Geometry: final body of the model. Coordinates: model frame, mm. Face numbers are marked on the shaded views. A direction names the side the tool comes from. Give positions to 0.01 mm unless a question says otherwise; leave off trailing zeros. Order: outer loops, then holes, each group sorted by start corner. A loop starts at its lowest first (then second) coordinate and runs counter-clockwise, first axis right, second up. Notation, with made-up numbers: (-25, -39) -> (-19, -39) arc R21 ccw to (-19, -21) -> close; hole circle Ø9 at (26.25, -31). An arc over 180 degrees is marked (long way). Answer in a Markdown table with one row per item. Add a question column.
Q1. Cut plane C-C on x = 13. Return the cut outline in (y, z).
Q2. Cut plane B-B on y = 9. Return the cut outline in (x, z), and give its area (3 significant figures).
Q3. Contact query for flat-ended pins moving along their axis: P1, Ø4, axis at y = 9.5, z = 11, coming from the -X side; P2, Ø8, axis at x = 13, y = 13, coming from the -Z side; P3, Ø1.2, axis at x = 18.5, z = 12, coming from the +Y side; P4, Ø3.5, axis at x = -13, y = 13, coming from the -Z side. Output: stop coordinate, or through.
Q4. Set-up query: the marked faces 1, 2, 3, 4 and 5. Return all of +Z, -Z, +X, -X, +Y, -Y with unobstructed straight access to the full face (end or side cutting, diameter ignored); none if empty.
Q5. Cut plane A-A on z = 8.5. Return the cut outline in (x, y).
Q6. Line query: line 1 along Y through (x, z) = (17.3, 8.5); line 2 along Y through (x, z) = (18.6, 8.5); line 3 along X through (y, z) = (-13, 3.9). Output: solid intervals per line, ascending. Write a range as from..to.
Q7. Cut plane D-D on x = -9. Return the cut outline in (y, z).
Q8. Pull-direction query (X, two-part tool) for the marked faces 6, 7, 8 and 9; classes: +X half, -X half, draft (parallel to the pull), parting line (faces both ways), or undercut.
from build123d import *

# Parameters (mm, degrees)
RESSALTO_EXTRUS_O1_DEPTH      = 4.5
CORTE_EXTRUS_O1_START         = -4.5
ESBO_O2_R                     = 5.1
CORTE_EXTRUS_O1_DEPTH         = 3.5
ESBO_O3_R                     = 3
CORTE_EXTRUS_O2_DEPTH         = 3.5
ESPELHAR2_COPY_1_DEPTH        = 4.5
ESPELHAR2_START               = -4.5
ESPELHAR2_COPY_2_SKETCH_R     = 5.1
ESPELHAR2_COPY_2_DEPTH        = 3.5
ESPELHAR2_COPY_3_SKETCH_R     = 3
ESPELHAR2_COPY_3_DEPTH        = 3.5
RESSALTO_EXTRUS_O2_START      = -3
ESBO_O5_W                     = 14
ESBO_O5_H                     = 14
RESSALTO_EXTRUS_O2_DEPTH      = 4
ESBO_O6_R                     = 5.15
CORTE_EXTRUS_O3_DEPTH         = 3.5
ESBO_O7_R                     = 3
CORTE_EXTRUS_O4_DEPTH         = 45.746508244
FILETE1_R                     = 10
RESSALTO_EXTRUS_O3_DEPTH      = 1
RESSALTO_EXTRUS_O3_DEPTH_BACK = 1
ESBO_O8_W                     = 8.485281374
ESBO_O8_H                     = 8
ESBO_O8_W_2                   = 9.485281374
ESPELHAR5_START               = -4.5
ESPELHAR5_COPY_1_SKETCH_R     = 5.1
ESPELHAR5_COPY_1_DEPTH        = 3.5
ESPELHAR5_COPY_2_SKETCH_R     = 5.1
ESPELHAR5_COPY_2_DEPTH        = 3.5


with BuildPart() as part:
    # Esboço1 → Ressalto-extrusão1 (new body)
    with BuildSketch(Plane.XY):
        Polygon((-8.485281374, 0), (-20, 11.514718626), (-20, 20), (-11.514718626, 20), (0, 8.485281374), (0, 0), align=None)
    ressalto_extrus_o1 = extrude(amount=RESSALTO_EXTRUS_O1_DEPTH)

    # Esboço2 → Corte-extrusão1 (cut)
    with BuildSketch(Plane.XY.offset(4.5).offset(CORTE_EXTRUS_O1_START)):
        with Locations((-13, 13)):
            Circle(ESBO_O2_R)
    corte_extrus_o1 = extrude(amount=CORTE_EXTRUS_O1_DEPTH, mode=Mode.SUBTRACT)

    # Esboço3 → Corte-extrusão2 (cut)
    with BuildSketch(Plane(origin=(0, 0, 3.5), x_dir=(-1, 0, 0), z_dir=(0, 0, -1))):
        with Locations((13, 13)):
            Circle(ESBO_O3_R)
    corte_extrus_o2 = extrude(amount=-CORTE_EXTRUS_O2_DEPTH, mode=Mode.SUBTRACT)

    # Espelhar1: Ressalto-extrusão1, Corte-extrusão1, Corte-extrusão2 across plane
    add(ressalto_extrus_o1.mirror(Plane(origin=(0, 0, 0), x_dir=(0, 0, 1), z_dir=(1, 0, 0))))
    add(corte_extrus_o1.mirror(Plane(origin=(0, 0, 0), x_dir=(0, 0, 1), z_dir=(1, 0, 0))), mode=Mode.SUBTRACT)
    add(corte_extrus_o2.mirror(Plane(origin=(0, 0, 0), x_dir=(0, 0, 1), z_dir=(1, 0, 0))), mode=Mode.SUBTRACT)

    # Espelhar2: Ressalto-extrusão1, Corte-extrusão1, Corte-extrusão2 across plane
    add(ressalto_extrus_o1.mirror(Plane.ZX))
    add(corte_extrus_o1.mirror(Plane.ZX), mode=Mode.SUBTRACT)
    add(corte_extrus_o2.mirror(Plane.ZX), mode=Mode.SUBTRACT)

    # Espelhar2 copy 1 sketch → Espelhar2 copy 1 (add)
    with BuildSketch(Plane(origin=(0, 0, 0), x_dir=(-1, 0, 0), z_dir=(0, 0, 1))):
        Polygon((-8.485281374, 0), (-20, 11.514718626), (-20, 20), (-11.514718626, 20), (0, 8.485281374), (0, 0), align=None)
    extrude(amount=ESPELHAR2_COPY_1_DEPTH)

    # Espelhar2 copy 2 sketch → Espelhar2 copy 2 (cut)
    with BuildSketch(Plane(origin=(0, 0, 4.5), x_dir=(-1, 0, 0), z_dir=(0, 0, 1)).offset(ESPELHAR2_START)):
        with Locations((-13, 13)):
            Circle(ESPELHAR2_COPY_2_SKETCH_R)
    extrude(amount=ESPELHAR2_COPY_2_DEPTH, mode=Mode.SUBTRACT)

    # Espelhar2 copy 3 sketch → Espelhar2 copy 3 (cut)
    with BuildSketch(Plane(origin=(0, 0, 3.5), x_dir=(1, 0, 0), z_dir=(0, 0, -1))):
        with Locations((13, 13)):
            Circle(ESPELHAR2_COPY_3_SKETCH_R)
    extrude(amount=-ESPELHAR2_COPY_3_DEPTH, mode=Mode.SUBTRACT)

    # Esboço5 → Ressalto-extrusão2 (add)
    with BuildSketch(Plane(origin=(20, 0, 0), x_dir=(0, 0, -1), z_dir=(1, 0, 0)).offset(RESSALTO_EXTRUS_O2_START)):
        with Locations((-7, 13)):
            Rectangle(ESBO_O5_W, ESBO_O5_H)
    ressalto_extrus_o2 = extrude(amount=RESSALTO_EXTRUS_O2_DEPTH)

    # Esboço6 → Corte-extrusão3 (cut)
    with BuildSketch(Plane.ZY.offset(-21)):
        with Locations((8.5, 13)):
            Circle(ESBO_O6_R)
    corte_extrus_o3 = extrude(amount=CORTE_EXTRUS_O3_DEPTH, mode=Mode.SUBTRACT)

    # Esboço7 → Corte-extrusão4 (cut, symmetric)
    with BuildSketch(Plane(origin=(17.5, 0, 0), x_dir=(0, 0, -1), z_dir=(1, 0, 0))):
        with Locations(Location((-8.5, 13, 0), (0, 0, 180))):
            Circle(ESBO_O7_R)
    corte_extrus_o4 = extrude(amount=CORTE_EXTRUS_O4_DEPTH, both=True, mode=Mode.SUBTRACT)

    # Espelhar3: Ressalto-extrusão2, Corte-extrusão3, Corte-extrusão4 across plane
    add(ressalto_extrus_o2.mirror(Plane.ZX))
    add(corte_extrus_o3.mirror(Plane.ZX), mode=Mode.SUBTRACT)
    add(corte_extrus_o4.mirror(Plane.ZX), mode=Mode.SUBTRACT)

    # Filete1
    # the kernel refuses this fillet: 10 mm, written as the material it adds along each edge
    with BuildSketch(Plane(origin=(17, 8.514718626, 4.5), x_dir=(0, -1, 0), z_dir=(0, 0, -1))) as filete1_piece_1:
        with BuildLine():
            CenterArc((12.353448055, -1.788687569), FILETE1_R, 135, 34.696124969)
            Line((5.282380243, 5.282380243), (0, 0))
            Line((0, 0), (2.514718626, 0))
        make_face()
    extrude(amount=4.5)
    with BuildSketch(Plane(origin=(17, -8.514718626, 0), x_dir=(-0.7071067811865464, 0.7071067811865487, 0), z_dir=(0, 0, 1))) as filete1_piece_2:
        with BuildLine():
            CenterArc((7.470413781, -10), FILETE1_R, 90, 34.696124969)
            Line((1.778174593, -1.778174593), (0, 0))
            Line((0, 0), (7.470413781, 0))
        make_face()
    extrude(amount=4.5)

    # Esboço8 → Ressalto-extrusão3 (add, two sides: drawn at the far end of the back side and taken through both)
    with BuildSketch(Plane(origin=(0, 20, 0), x_dir=(1, 0, 0), z_dir=(0, 1, 0)).offset(-RESSALTO_EXTRUS_O3_DEPTH_BACK)):
        with Locations((-15.757359313, -4)):
            Rectangle(ESBO_O8_W, ESBO_O8_H)
        with Locations((16.257359313, -4)):
            Rectangle(ESBO_O8_W_2, ESBO_O8_H)
    extrude(amount=RESSALTO_EXTRUS_O3_DEPTH + RESSALTO_EXTRUS_O3_DEPTH_BACK)

    # Espelhar4: Corte-extrusão1 across plane
    add(corte_extrus_o1.mirror(Plane(origin=(0, 0, 0), x_dir=(0, 0, 1), z_dir=(1, 0, 0))), mode=Mode.SUBTRACT)

    # Espelhar5 copy 1 sketch → Espelhar5 copy 1 (cut)
    with BuildSketch(Plane(origin=(0, 0, 4.5), x_dir=(-1, 0, 0), z_dir=(0, 0, 1)).offset(ESPELHAR5_START)):
        with Locations((-13, 13)):
            Circle(ESPELHAR5_COPY_1_SKETCH_R)
    extrude(amount=ESPELHAR5_COPY_1_DEPTH, mode=Mode.SUBTRACT)

    # Espelhar5 copy 2 sketch → Espelhar5 copy 2 (cut)
    with BuildSketch(Plane.XY.offset(4.5).offset(ESPELHAR5_START)):
        with Locations((-13, -13)):
            Circle(ESPELHAR5_COPY_2_SKETCH_R)
    extrude(amount=ESPELHAR5_COPY_2_DEPTH, mode=Mode.SUBTRACT)


solid = part.part
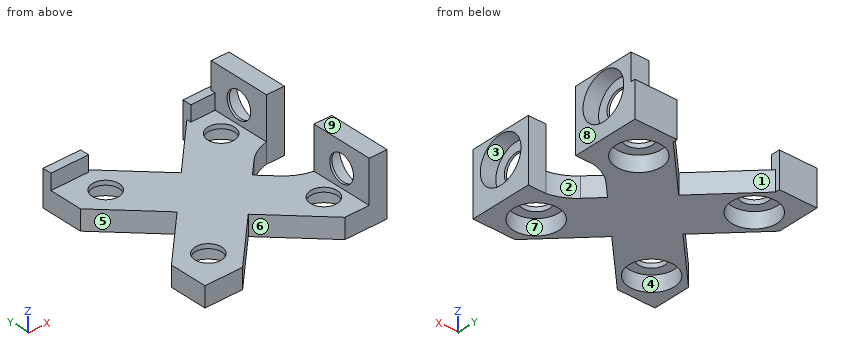
Completed:
| question | item | result |
|---|---|---|
| 1 | outline | (-20, 0) -> (-18.1, 0) -> (-18.1, 3.5) -> (-16, 3.5) -> (-16, 4.5) -> (-20, 4.5) -> close; (-10, 3.5) -> (-7.9, 3.5) -> (-7.9, 0) -> (-4.32, 0) -> (-4.32, 4.5) -> (-10, 4.5) -> close; (4.32, 0) -> (7.9, 0) -> (7.9, 3.5) -> (10, 3.5) -> (10, 4.5) -> (4.32, 4.5) -> close; (16, 3.5) -> (18.1, 3.5) -> (18.1, 0) -> (21, 0) -> (21, 8) -> (19, 8) -> (19, 4.5) -> (16, 4.5) -> close |
| 2 | outline | (-17.49, 0) -> (-16.16, 0) -> (-16.16, 3.5) -> (-9.84, 3.5) -> (-9.84, 0) -> (-0.51, 0) -> (-0.51, 4.5) -> (-17.49, 4.5) -> close; (0.51, 0) -> (9.84, 0) -> (9.84, 3.5) -> (16.16, 3.5) -> (16.16, 0) -> (21, 0) -> (21, 5.26) -> (17.5, 5.26) -> (17.5, 11.74) -> (21, 11.74) -> (21, 14) -> (17, 14) -> (17, 4.5) -> (0.51, 4.5) -> close |
| 2 | area | 140 mm² |
| 3 | P1 | stops at x = 17 |
| 3 | P2 | stops at z = 3.5 |
| 3 | P3 | stops at y = 20 |
| 3 | P4 | passes through |
| 4 | face 1 | +Z, -Z, +Y |
| 4 | face 2 | +Z, -Z, +X |
| 4 | face 3 | +X |
| 4 | face 4 | -Z |
| 4 | face 5 | +Z, -Z, -X |
| 5 | outline | (17, -20) -> (21, -20) -> (21, -18.15) -> (17.5, -18.15) -> (17.5, -16) -> (17, -16) -> close; (17, -10) -> (17.5, -10) -> (17.5, -7.85) -> (21, -7.85) -> (21, -6) -> (17, -6) -> close; (17, 6) -> (21, 6) -> (21, 7.85) -> (17.5, 7.85) -> (17.5, 10) -> (17, 10) -> close; (17, 16) -> (17.5, 16) -> (17.5, 18.15) -> (21, 18.15) -> (21, 20) -> (17, 20) -> close |
| 6 | line 1 | y = -20..-16, -10..-6, 6..10, 16..20 |
| 6 | line 2 | y = -20..-18.15, -7.85..-6, 6..7.85, 18.15..20 |
| 6 | line 3 | x = -20..-16, -10..-4.51, 4.51..10, 16..17.5 |
| 7 | outline | (-17.49, 0) -> (-16.16, 0) -> (-16.16, 3.5) -> (-9.84, 3.5) -> (-9.84, 0) -> (-0.51, 0) -> (-0.51, 4.5) -> (-17.49, 4.5) -> close; (0.51, 0) -> (9.84, 0) -> (9.84, 3.5) -> (16.16, 3.5) -> (16.16, 0) -> (17.49, 0) -> (17.49, 4.5) -> (0.51, 4.5) -> close |
| 8 | face 6 | undercut |
| 8 | face 7 | undercut |
| 8 | face 8 | +X half |
| 8 | face 9 | draft |
